The listing builds one solid part. Answer for the finished solid, in the listing's coordinates (mm). A direction names the side the tool comes from. Coordinates: 2 decimals unless noted, no trailing zeros. Order: outer loops, then holes, each group sorted by start corner. A loop starts at its lowest first (then second) coordinate and runs counter-clockwise, first axis right, second up. Notation, with made-up numbers: (65.5, 84.5) - (124.5, 84.5) arc R23 cw to (124.5, 115.5) - close; hole circle Ø9 at (85, 8.5). An arc over 180 degrees is marked (long way). Use one line per item in the form item = value. Start each with the question number.
Item 1: A tool of negligible diameter and unlimited length cuts with its end or side. For faces 1 (the flat face through (-2, 9, 1.5)), 2 (the flat face through (5, 9.352, 1)), 3 (the cylindrical face through (-2.93, -0.31, 1.86)), from which of +Z, -Z, +X, -X, +Y, -Y can it reach the whole face along a straight path? Write none if from no direction.
Item 2: Section B-B, the plane z = 1.7 is taken. Write down the section's boundary in (x, y), and give its area (3 significant figures).
Item 3: Consider line 1 along Z through (x, y) = (4.75, -0.5); line 2 along X through (y, z) = (8.5, 0.75); line 3 along X through (y, z) = (7.75, 0.65) (3 decimals). Determine where each line is inside the solid, lowest interval first. Write a range as [from, to].
Item 4: Section A-A, the plane z = 0.7 is taken. Write down the section's boundary in (x, y), and give its area (3 significant figures).
from build123d import *

# Parameters (mm, degrees)
F1_DEPTH = 1.5
F2_R     = 1
F3_R     = 1
F5_DEPTH = 0.5
F6_R     = 0.49999


# Not quite as in the source:
# - a fillet or chamfer is up to 0.001 mm smaller than in the source, because OpenCascade refuses the exact size


with BuildPart() as f1:
    # F0 (on Top) → F1 (new body)
    with BuildSketch(Plane.XY):
        with BuildLine():
            ThreePointArc((-1.986540854, 9.3519296497), (0, 10.2135319331), (1.986540854, 9.3519296497))
            Line((1.986540854, 9.3519296497), (3.4759494504, 9.3519296497))
            ThreePointArc((3.4759494504, 9.3519296497), (0, 11.4346017651), (-3.4759494504, 9.3519296497))
            Line((-3.4759494504, 9.3519296497), (-1.986540854, 9.3519296497))
        make_face()
        with BuildLine():
            Line((5.9530865401, 9.3519296497), (3.4759494504, 9.3519296497))
            ThreePointArc((3.4759494504, 9.3519296497), (3.8237056455, 8.4510290854), (3.9419905804, 7.4926111847))
            ThreePointArc((3.9419905804, 7.4926111847), (-0.9584179006, 3.6689055392), (-3.4759494504, 9.3519296497))
            Line((-3.4759494504, 9.3519296497), (-5.9530865401, 9.3519296497))
            Line((-5.9530865401, 9.3519296497), (-7.8950412571, 7.5339297764))
            Line((-7.8950412571, 7.5339297764), (-8.927995339, 4.88956552))
            Line((-8.927995339, 4.88956552), (-7.4818595313, 1.1296109296))
            Line((-7.4818595313, 1.1296109296), (0, -4.9441619776))
            Line((0, -4.9441619776), (7.4818595313, 1.1296109296))
            Line((7.4818595313, 1.1296109296), (8.927995339, 4.88956552))
            Line((8.927995339, 4.88956552), (7.8950412571, 7.5339297764))
            Line((7.8950412571, 7.5339297764), (5.9530865401, 9.3519296497))
        make_face()
        with BuildLine():
            Line((3.4759494504, 9.3519296497), (1.986540854, 9.3519296497))
            ThreePointArc((1.986540854, 9.3519296497), (2.5306748058, 8.4921584552), (2.7209207483, 7.4926111847))
            ThreePointArc((2.7209207483, 7.4926111847), (-0.9995472705, 4.9619363789), (-1.986540854, 9.3519296497))
            Line((-1.986540854, 9.3519296497), (-3.4759494504, 9.3519296497))
            ThreePointArc((-3.4759494504, 9.3519296497), (-0.9584179006, 3.6689055392), (3.9419905804, 7.4926111847))
            ThreePointArc((3.9419905804, 7.4926111847), (3.8237056455, 8.4510290854), (3.4759494504, 9.3519296497))
        make_face()
        with BuildLine():
            Line((1.986540854, 9.3519296497), (0, 7.4926111847))
            Line((0, 7.4926111847), (-1.986540854, 9.3519296497))
            ThreePointArc((-1.986540854, 9.3519296497), (-0.9995472705, 4.9619363789), (2.7209207483, 7.4926111847))
            ThreePointArc((2.7209207483, 7.4926111847), (2.5306748058, 8.4921584552), (1.986540854, 9.3519296497))
        make_face()
    extrude(amount=F1_DEPTH)

    # F2
    f2_edges = [f1.edges().sort_by_distance(p)[0] for p in [
        (0, -4.944162, 0.75),
    ]]
    fillet(f2_edges, radius=F2_R)

    # F3
    f3_edges = [f1.edges().sort_by_distance(p)[0] for p in [
        (7.48186, 1.129611, 0.75),
        (8.927995, 4.889566, 0.75),
        (7.895041, 7.53393, 0.75),
        (5.953087, 9.35193, 0.75),
        (-7.48186, 1.129611, 0.75),
        (-8.927995, 4.889566, 0.75),
        (-7.895041, 7.53393, 0.75),
        (-5.953087, 9.35193, 0.75),
        (-3.475949, 9.35193, 0.75),
        (3.475949, 9.35193, 0.75),
    ]]
    fillet(f3_edges, radius=F3_R)

    # F4 (on face) → F5 (join)
    with BuildSketch(Plane.XY.offset(1.5)):
        with BuildLine():
            ThreePointArc((-1.7098843542, 9.0929908328), (-1.8141917234, 8.9737012946), (-1.9101937031, 8.8476313097))
            ThreePointArc((-1.9101937031, 8.8476313097), (-2.837339859, 8.0420404539), (-4.0308273111, 7.7519295737))
            Line((-4.0308273111, 7.7519295737), (-5.3210256953, 7.7519295737))
            Line((-5.3210256953, 7.7519295737), (-6.5367130105, 6.613839501))
            Line((-6.5367130105, 6.613839501), (-7.2120080925, 4.88508291))
            Line((-7.2120080925, 4.88508291), (-6.141831705, 2.1026231998))
            Line((-6.141831705, 2.1026231998), (0, -2.8833152363))
            Line((0, -2.8833152363), (6.141831705, 2.1026231998))
            Line((6.141831705, 2.1026231998), (7.2120080925, 4.88508291))
            Line((7.2120080925, 4.88508291), (6.5367130105, 6.613839501))
            Line((6.5367130105, 6.613839501), (5.3210256953, 7.7519295737))
            Line((5.3210256953, 7.7519295737), (4.0308273111, 7.7519295737))
            ThreePointArc((4.0308273111, 7.7519295737), (2.837339859, 8.0420404539), (1.9101937031, 8.8476313097))
            ThreePointArc((1.9101937031, 8.8476313097), (1.8141917234, 8.9737012946), (1.7098843542, 9.0929908328))
            Line((1.7098843542, 9.0929908328), (0, 7.4926111847))
            Line((0, 7.4926111847), (-1.7098843542, 9.0929908328))
        make_face()
    extrude(amount=F5_DEPTH)

    # F6 (radius 0.5 in the source; OpenCascade refuses exactly that, so slightly less here)
    f6_edges = [f1.edges().sort_by_distance(p)[0] for p in [
        (-5.928869, 7.182885, 2),
        (-6.874361, 5.749461, 2),
        (-6.67692, 3.493853, 2),
        (-3.070916, -0.390346, 2),
        (3.070916, -0.390346, 2),
        (6.67692, 3.493853, 2),
        (6.874361, 5.749461, 2),
        (5.928869, 7.182885, 2),
        (4.675927, 7.75193, 2),
        (2.83734, 8.04204, 2),
        (-2.83734, 8.04204, 2),
    ]]
    fillet(f6_edges, radius=F6_R)


solid = f1.part
Response:
q1.face_1 = +Z
q1.face_2 = +Z, -Z, +X, +Y
q1.face_3 = +Z, -X, -Y
q2.outline = (-7.17, 4.88) - (-6.11, 2.13) - (0, -2.83) - (6.11, 2.13) - (7.17, 4.88) - (6.5, 6.59) - (5.3, 7.71) - (4.03, 7.71) arc R2.64 cw to (1.88, 8.82) arc R2.3 ccw to (1.68, 9.06) - (0, 7.49) - (-1.68, 9.06) arc R2.3 ccw to (-1.88, 8.82) arc R2.64 cw to (-4.03, 7.71) - (-5.3, 7.71) - (-6.5, 6.59) - close
q2.area = 107 mm2
q3.line_1 = [0, 1.5]
q3.line_2 = [-6.86, -1.08], [1.08, 6.86]
q3.line_3 = [-7.664, -0.275], [0.275, 7.664]
q4.outline = (-8.79, 4.53) - (-7.58, 1.38) arc R1 ccw to (-7.27, 0.96) - (-0.63, -4.43) arc R1 ccw to (0.63, -4.43) - (7.27, 0.96) arc R1 ccw to (7.58, 1.38) - (8.79, 4.53) arc R1 ccw to (8.79, 5.25) - (7.98, 7.32) arc R1 ccw to (7.73, 7.69) - (6.24, 9.08) arc R1 ccw to (5.56, 9.35) - (4.03, 9.35) arc R1 cw to (3.22, 9.77) arc R3.94 ccw to (-3.22, 9.77) arc R1 cw to (-4.03, 9.35) - (-5.56, 9.35) arc R1 ccw to (-6.24, 9.08) - (-7.73, 7.69) arc R1 ccw to (-7.98, 7.32) - (-8.79, 5.25) arc R1 ccw to start; hole (-1.99, 9.35) - (0, 7.49) - (1.99, 9.35) arc R2.72 ccw to start
q4.area = 181 mm2
